Build history of the part. All positions in model axes, mm. A direction names the side the tool comes from. Round coordinates to 2 decimals unless told otherwise and drop trailing zeros. Write each loop counter-clockwise with the first axis right and the second up, starting at its lowest first coordinate (ties: lowest second). Pieces come first, ordered by that corner, then holes. Notation, with made-up numbers: (-27.5, 48.25) - (-17.5, 48.25) arc R19 ccw to (-17.5, 72.25) - close; hole circle Ø6 at (72.25, -1). An arc over 180 degrees is marked (long way). Write each question's results on one line, items separated by ' | '.
Solid Edge part; units mm, degrees
sketch "Sketch1" plane through (0, 0, 0) normal (0, -1, 0) x (1, 0, 0)
  line L0 (-40, -15) -> (-36, -15)
  line L1 (-36, -15) -> (-36, -4)
  line L2 (-36, -4) -> (36, -4)
  line L3 (36, -4) -> (36, -15)
  line L4 (36, -15) -> (40, -15)
  line L5 (40, -15) -> (40, 0)
  line L6 (40, 0) -> (-40, 0)
  line L7 (-40, 0) -> (-40, -15)
  dimension "D1" = 40
  dimension "D2" = 40
  dimension "D3" = 40
extrude "v_1_body" add sketch "Sketch1" against normal blind 75 and the other way blind 75
fillet "v_1_side_rounds" radius 4 4 edges at (36, 0, -4) (-36, 0, -4) (40, 0, 0) (-40, 0, 0)
hole "Hole1" at (-20, 40, 0) direction (0, 0, -1) diameter 16 end up to next start chamfer 1.1 start chamfer angle 45 end chamfer 1.1 end chamfer angle 45
hole "Hole2" at (-20, 10, 0) direction (0, 0, -1) diameter 16 end up to next start chamfer 1.1 start chamfer angle 45 end chamfer 1.1 end chamfer angle 45
hole "Hole3" at (-20, -20, 0) direction (0, 0, -1) diameter 16 end up to next start chamfer 1.1 start chamfer angle 45 end chamfer 1.1 end chamfer angle 45
hole "Hole4" at (15, -30, 0) direction (0, 0, -1) diameter 16 end up to next start chamfer 1.1 start chamfer angle 45 end chamfer 1.1 end chamfer angle 45
sketch "Sketch2" plane through (0, 0, 0) normal (0, 0, 1) x (1, 0, 0)
  line L0 (6, 35) -> (26, 35)
  line L1 (26, 35) -> (26, 10)
  line L2 (26, 10) -> (6, 10)
  line L3 (6, 10) -> (6, 35)
extrude "Cutout1" cut sketch "Sketch2" against normal up to next
extrude "v_1_ult_cap_bearing_bodies" [suppressed]
fillet "v_1_ult_cap_bearing_counds" [suppressed]
hole "v_1_ult_cap_hole" [suppressed]
properties material "Polypropylene, general purpose"
(1) Tool access for faces 4 (the flat face through (16, 10, -2)), 5 (the cylindrical face through (34.859, -1.05, -5.203)), 6 (the flat face through (-38, -1, -15)): list every direction of +Z, -Z, +X, -X, +Y, -Y with a clear straight run to the whole face (end or side of a thin tool).
Worked answers:
face 4: +Z, -Z | face 5: -Z, +Y, -Y | face 6: -Z, +X, -X, +Y, -Y
(2) Slice it at A-A, the plane x = 15. Write the cut outline in (y, z).
Worked answers:
outline: (-75, -4) - (-39.1, -4) - (-38, -2.9) - (-38, -1.1) - (-39.1, 0) - (-75, 0) - close; (-22, -2.9) - (-20.9, -4) - (10, -4) - (10, 0) - (-20.9, 0) - (-22, -1.1) - close; (35, -4) - (75, -4) - (75, 0) - (35, 0) - close
(3) Two-plate mould, pull along Y, no slides. Class faces 1 (the flat face through (0, -75, -2)), 2 (the cylindrical face through (-38.859, 1.05, -1.203)), 3 (the flat face through (16, 35, -2)): released by +Y, released by -Y, zero draft, split by the parting line, or undercut.
Worked answers:
face 1: released by -Y | face 2: zero draft | face 3: undercut
(4) Drill centre lines: probe 1 along Y at (x, z) = (-20, -1.55); probe 2 along X at (y, z) = (-4, -11.5); probe 3 along Z at (x, y) = (-6, 15). Where is each one in solid material? Low to high. Write a range as [from, to].
Worked answers:
probe 1: y = [-75, -28], [-12, 2], [18, 32], [48, 75] | probe 2: x = [-40, -36], [36, 40] | probe 3: z = [-4, 0]
(5) Slice it at C-C, the plane z = -13.25. Write the cut outline in (x, y).
Worked answers:
outline: (-40, -75) - (-36, -75) - (-36, 75) - (-40, 75) - close; (36, -75) - (40, -75) - (40, 75) - (36, 75) - close
(6) Slice it at D-D, the plane x = -20. Write the cut outline in (y, z).
Worked answers:
outline: (-75, -4) - (-29.1, -4) - (-28, -2.9) - (-28, -1.1) - (-29.1, 0) - (-75, 0) - close; (-12, -2.9) - (-10.9, -4) - (0.9, -4) - (2, -2.9) - (2, -1.1) - (0.9, 0) - (-10.9, 0) - (-12, -1.1) - close; (18, -2.9) - (19.1, -4) - (30.9, -4) - (32, -2.9) - (32, -1.1) - (30.9, 0) - (19.1, 0) - (18, -1.1) - close; (48, -2.9) - (49.1, -4) - (75, -4) - (75, 0) - (49.1, 0) - (48, -1.1) - close
(7) Slice it at B-B, the plane y = 40. Write the cut outline in (x, z).
Worked answers:
outline: (-40, -15) - (-36, -15) - (-36, -8) arc R4 cw to (-32, -4) - (-29.1, -4) - (-28, -2.9) - (-28, -1.1) - (-29.1, 0) - (-36, 0) arc R4 ccw to (-40, -4) - close; (-12, -2.9) - (-10.9, -4) - (32, -4) arc R4 cw to (36, -8) - (36, -15) - (40, -15) - (40, -4) arc R4 ccw to (36, 0) - (-10.9, 0) - (-12, -1.1) - close
(8) Flat gauge pins, fed straight in: pin 1 Ø3 at (y, z) = (-34, -2) entering from -X; pin 2 Ø3 at (y, z) = (20.5, -1) entering from -X; pin 3 Ø21 at (x, y) = (15, -30) entering from +Z; pin 4 Ø19 at (x, y) = (-12, 30) entering from -Z. Where does each tip first touch, or does it go through?
Worked answers:
pin 1: stops at x = -39.97 | pin 2: stops at x = -39.71 | pin 3: stops at z = 0 | pin 4: stops at z = -4
